Read the model definition and answer for the solid it produces. Units are mm, in the model's axes. A direction names the side the tool comes from. Coordinates: 2 decimals unless noted, no trailing zeros. Order: outer loops, then holes, each group sorted by start corner. A loop starts at its lowest first (then second) coordinate and runs counter-clockwise, first axis right, second up. Notation, with made-up numbers: (63.5, 27.25) - (75.5, 27.25) arc R14 ccw to (75.5, 43.25) - close; hole circle Ø5 at (87, 73.25). An arc over 180 degrees is marked (long way). Use one line per item in the form item = value. Start each with the question number.
from build123d import *

# Parameters (mm, degrees)
F0_W     = 140
F0_H     = 140
F0_W_2   = 40
F0_H_2   = 130
F1_DEPTH = 25
F2_DEPTH = 35
F3_R     = 10
F4_R     = 5


with BuildPart() as f1:
    # F0 (on Top) → F1 (new body)
    with BuildSketch(Plane.XY):
        Rectangle(F0_W, F0_H)
        Rectangle(F0_W_2, F0_H_2, mode=Mode.SUBTRACT)
    extrude(amount=F1_DEPTH)

    # F0 (on Top) → F2 (join)
    with BuildSketch(Plane.XY):
        Rectangle(F0_W_2, F0_H_2)
    extrude(amount=F2_DEPTH)

    # F3
    f3_edges = [f1.edges().sort_by_distance(p)[0] for p in [
        (-70, 70, 12.5),
        (70, 70, 12.5),
        (70, -70, 12.5),
        (-70, -70, 12.5),
    ]]
    fillet(f3_edges, radius=F3_R)

    # F4
    f4_edges = [f1.edges().sort_by_distance(p)[0] for p in [
        (-20, -65, 30),
        (20, -65, 30),
        (20, 65, 30),
        (-20, 65, 30),
    ]]
    fillet(f4_edges, radius=F4_R)


solid = f1.part
Q1. Consider probe 1 along Z at (x, y) = (-21.5, 3); probe 2 along Y at (x, z) = (-10.5, 27); probe 3 along X at (y, z) = (-13, 30). Determine where each line is inside the solid, lowest interval first.
Q2. A cutting plane is placed at B-B (y = -47.5). Give the vertices of the cut face in (x, z).
Q3. Which of the six approach directions +Z, -Z, +X, -X, +Y, -Y give full straight-line access (tool end or side, diameter ignored) to faces 1 (the flat face through (20, -1, 30)), 2 (the cylindrical face through (19, 63, 30)), 3 (the flat face through (0, 65, 30)), 4 (the cylindrical face through (-18, -64, 30))?
Q4. A cutting plane is placed at A-A (x = 4). Give the vertices of the cut face in (y, z).
Q5. Given P1, Ø5, axis at x = -35.5, y = -34.5, coming from the +Z side; P2, Ø8, axis at x = 3.5, z = 29.5, coming from the +Y side; P3, Ø3, axis at x = -0.5, z = 30, coming from the -Y side, each flat-ended and moving along its own axis, determine where each tip first touches the part or whether it passes through.
Q6. A cutting plane is placed at C-C (x = 47). Give the vertices of the cut face in (y, z).
Result sheet:
q1.probe_1 = 0 to 25
q1.probe_2 = -65 to 65
q1.probe_3 = -20 to 20
q2.outline = (-70, 0) - (70, 0) - (70, 25) - (20, 25) - (20, 35) - (-20, 35) - (-20, 25) - (-70, 25) - close
q3.face_1 = +Z, +X, +Y, -Y
q3.face_2 = +Z, +X, +Y
q3.face_3 = +Z, +X, -X, +Y
q3.face_4 = +Z, -X, -Y
q4.outline = (-70, 0) - (70, 0) - (70, 25) - (65, 25) - (65, 35) - (-65, 35) - (-65, 25) - (-70, 25) - close
q5.P1 = 25
q5.P2 = 65
q5.P3 = -65
q6.outline = (-70, 0) - (70, 0) - (70, 25) - (-70, 25) - close
